Read the model definition and answer for the solid it produces. Units are mm, in the model's axes. Face numbers are marked on the shaded views. A direction names the side the tool comes from. Give positions to 0.01 mm unless a question says otherwise; leave off trailing zeros. Order: outer loops, then holes, each group sorted by start corner. A loop starts at its lowest first (then second) coordinate and runs counter-clockwise, first axis right, second up. Notation, with made-up numbers: (48, -24) -> (90, -24) arc R17 ccw to (90, -10) -> close; hole circle Ø4 at (-22, 28). An arc over 180 degrees is marked (long way). Use one line per item in the form item = value.
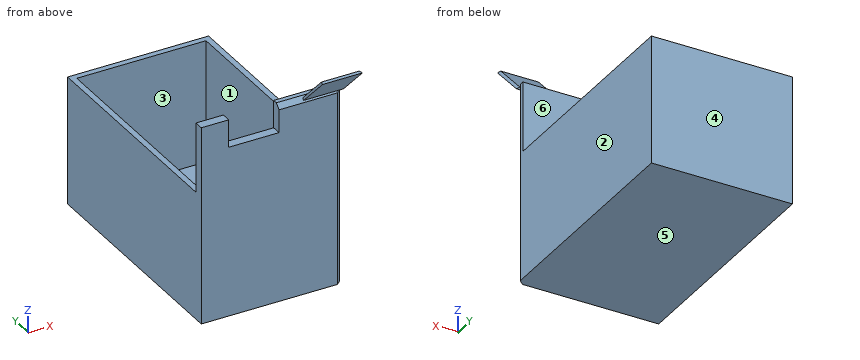
```python
from build123d import *

# Parameters (mm, degrees)
F0_W         = 76.2
F0_H         = 127
F1_DEPTH     = 69.342
F3_DEPTH     = 5.08
F4_T         = -3.175
F7_SIZE      = 2.54
F8_W         = 25.4
F8_H         = 1.27
F9_DEPTH     = 25.4
F10_T1_DEPTH = 38.4641495789


# Not quite as in the source:
# - a fillet or chamfer that OpenCascade refuses, or shapes differently, is made with other operations: its cross-section is extruded or revolved along the edge and cut away or added
# - a feature of the source that left no trace in its solid (it failed there, or was rolled back) is left out


with BuildPart() as f1:
    # F0 (on Top) → F1 (new body)
    with BuildSketch(Plane.XY):
        with Locations((38.1, 63.5)):
            Rectangle(F0_W, F0_H)
    extrude(amount=F1_DEPTH)

    # F2 (on face) → F3 (join)
    with BuildSketch(Plane.XZ):
        Polygon((0, 107.1759281516), (0, 69.342), (76.2, 69.342), (76.2, 107.1759281516), (42.011950165, 107.1759281516), (42.011950165, 92.1983985066), (14.8228770122, 92.1983985066), (14.8228770122, 107.1759281516), align=None)
    extrude(amount=-F3_DEPTH)

    # F4: a shell. OpenCascade refuses it in one call, so the cavity is built on its own and cut out:
    # the body offset inwards by the wall thickness, plus a prism from it out through each open face.
    f4_core = offset(f1.part, amount=F4_T, kind=Kind.INTERSECTION, mode=Mode.PRIVATE)
    f4_exits = [f4_core.faces().sort_by_distance(p)[0] for p in [
        (38.1, 63.5, 66.167),
    ]]
    add(f4_core, mode=Mode.SUBTRACT)
    extrude(f4_exits, amount=-F4_T, mode=Mode.SUBTRACT)

    # F7
    f7_edges = [f1.edges().sort_by_distance(p)[0] for p in [
        (59.105975, 0, 107.175928),
        (76.2, 0, 53.587964),
    ]]
    chamfer(f7_edges, length=F7_SIZE)

    # F8 (on face) → F9 (join)
    with BuildSketch(Plane(origin=(0, -52.3179640758, 52.3179640758), x_dir=(1, 0, 0), z_dir=(0, -0.7071067812, 0.7071067812))):
        with Locations((68.3882001948, 75.6758768002)):
            Rectangle(F8_W, F8_H)
    extrude(amount=F9_DEPTH)

    # F10: chamfer of 5.08 on 1 edges, made by hand

    # F10_s2 → F10_t1 (cut)
    with BuildSketch(Plane(origin=(0, -52.3179640758, 52.3179640758), x_dir=(1, 0, 0), z_dir=(0, -0.7071067812, 0.7071067812))):
        Polygon((76.0082001948, 76.3108768002), (81.0882001948, 71.2308768002), (81.0882001948, 76.3108768002), align=None)
    extrude(amount=F10_T1_DEPTH, mode=Mode.SUBTRACT)


solid = f1.part
```
Item 1: Which of the six approach directions +Z, -Z, +X, -X, +Y, -Y give full straight-line access (tool end or side, diameter ignored) to the marked faces 5 and 6?
Checks:
face_5 = -Z, +X, -X, +Y, -Y
face_6 = +Z, +X, -X, +Y
Item 2: Straight lines are drawn through the part: L1, parallel to Y at x = 66.5, z = 49.5 (3 decimals); L2, parallel to X at y = 105, z = 20 (3 decimals); L3, parallel to Z at x = 14, y = 9.5 (3 decimals). For each, find the intervals that lie inside material, in ascending order. Write a range as from..to.
Checks:
L1 = 0..3.175, 123.825..127
L2 = 0..3.175, 73.025..76.2
L3 = 0..3.175
Item 3: The part is cut by section C-C on y = 81.5. Give the vertices of the cut face in (x, z) (3 decimals), and give its area (3 significant figures).
Checks:
outline = (0, 0) -> (76.2, 0) -> (76.2, 69.342) -> (73.025, 69.342) -> (73.025, 3.175) -> (3.175, 3.175) -> (3.175, 69.342) -> (0, 69.342) -> close
area = 662 mm²
Item 4: The part is cut by section A-A on z = 37. Give the vertices of the cut face in (x, y) (3 decimals).
Checks:
outline = (0, 0) -> (73.66, 0) -> (76.2, 2.54) -> (76.2, 127) -> (0, 127) -> close; hole (3.175, 3.175) -> (73.025, 3.175) -> (73.025, 123.825) -> (3.175, 123.825) -> close
Item 5: The part is cut by section D-D on x = 23.5. Give the vertices of the cut face in (y, z) (3 decimals).
Checks:
outline = (0, 0) -> (127, 0) -> (127, 69.342) -> (123.825, 69.342) -> (123.825, 3.175) -> (3.175, 3.175) -> (3.175, 69.342) -> (5.08, 69.342) -> (5.08, 92.198) -> (0, 92.198) -> close
Item 6: Given pin 1 Ø8 at (x, y) = (14, 110.5) entering from +Z (3 decimals); pin 2 Ø11.5 at (x, z) = (30, 80.5) entering from +Y; pin 3 Ø5 at (y, z) = (18, 15.5) entering from +X, each flat-ended and moving along its own axis, determine where each tip first touches the part or whether it passes through.
Checks:
pin_1 = 3.175
pin_2 = 5.08
pin_3 = 76.2
Item 7: The part is cut by section B-B on x = 52.5. Give the vertices of the cut face in (y, z) (3 decimals).
Checks:
outline = (0, 0) -> (127, 0) -> (127, 69.342) -> (123.825, 69.342) -> (123.825, 3.175) -> (3.175, 3.175) -> (3.175, 69.342) -> (5.08, 69.342) -> (5.08, 107.176) -> (2.54, 107.176) -> (0, 104.636) -> close
Item 8: Determine the mould class of the marked faces 1, 2, 3 and 4 for opening direction Y: +Y half, -Y half, draft (parallel to the pull), parting line (faces both ways), or undercut.
Checks:
face_1 = undercut
face_2 = draft
face_3 = undercut
face_4 = +Y half
